Autodesk Inventor part; units mm, degrees
ref_plane "YZ Plane" through (0, 0, 0) normal (1, 0, 0) x (0, 1, 0)
ref_plane "XZ Plane" through (0, 0, 0) normal (0, 1, 0) x (-1, 0, 0)
ref_plane "XY Plane" through (0, 0, 0) normal (0, 0, 1) x (1, 0, 0)
sketch "Sketch1" plane through (0, 0, 0) normal (0, 0, 1) x (1, 0, 0)
  line L0 (0, -12.5) -> (0, 12.5)
  line L1 (9, 12.5) -> (9, -12.5)
  line L2 (9, -12.5) -> (4, -12.5)
  line L3 (4, -12.5) -> (4, 5.5)
  line L4 (4, 5.5) -> (2.5, 5.5)
  line L5 (2.5, 5.5) -> (2.5, 12.5)
  line L6 (2.5, 12.5) -> (9, 12.5)
  point P0 (0, 0)
  point P1 (0, 0)
  dimension "d0" = 18
  dimension "d1" = 25
  dimension "d2" = 8
  dimension "d3" = 5
  dimension "d4" = 18
revolve "Revolution1" add sketch "Sketch1" angle 360 about axis through (0, -12.5, 0) along (0, 1, 0)
sketch "Sketch2" plane through (0, 0, 0) normal (1, 0, 0) x (0, 1, 0)
  line L0 (12.5, -2.5) -> (12.5, 2.5)
  line L1 (-12.5, -4) -> (-12.5, 4)
  point P0 (0, 0)
  point P1 (9, 0)
  point P2 (-9, 0)
  dimension "d6" = 3.5
  dimension "d7" = 3.5
hole "Hole1" at (0, 9, 0) at (0, -9, 0) direction (-1, 0, 0) diameter 3.242 end through all
chamfer "Chamfer1" distance 0.3 angle 45 4 edges at (-9, 12.5, 0) (-2.5, 12.5, 0) (-9, -12.5, 0) (-4, -12.5, 0)
pattern_circular "Circular Pattern1" count 2 over 90 about axis through (0, 0, 0) along (0, 1, 0) of "Hole1"
properties part number "spring-shaft-coupler" material "Aluminum 6061-AHC"
Can you work these out from the model? Positions are in its coordinate system, mm. A direction names the side the tool comes from. Give positions to 0.01 mm unless a question says otherwise; leave off trailing zeros. Loops run counter-clockwise (first coordinate to the right, second up) from the corner with the lowest first, then second, coordinate; pieces in that order, holes last. Notation, with made-up numbers: (70, 43.25) - (90, 43.25) arc R23 ccw to (90, 56.25) - close; hole circle Ø6 at (78.25, -37.5). An arc over 180 degrees is marked (long way). Answer as a JSON object with one key per item and string values.
Q1. If we mould it in two halves opening along X, with no side actions, what happens to faces 1 (the cylindrical face through (1.34, 8.9, -2.11)), 2 (the cylindrical face through (-6.366, -7.562, -0.748)), 3 (the cylindrical face through (4.153, -0.171, -7.985))? For each: pulls with the +X half, pulls with the -X half, needs draft (parallel to the pull), parting line crosses it, or undercut.
Geometry says:
{"face 1": "undercut", "face 2": "needs draft", "face 3": "parting line crosses it"}
Q2. Imagine slicing it at D-D on y = -5. Write out the boundary of the cut face in (x, z).
Geometry says:
{"outline": "circle Ø18 at (0, 0); hole circle Ø8 at (0, 0)"}
Q3. Imagine slicing it at B-B on z = 0. Write out the boundary of the cut face in (x, y), plus the area to 3 significant figures.
Geometry says:
{"outline": "(-9, -12.2) - (-8.7, -12.5) - (-4.3, -12.5) - (-4, -12.2) - (-4, -10.62) - (-9, -10.62) - close; (-9, -7.38) - (-4, -7.38) - (-4, 5.5) - (-2.5, 5.5) - (-2.5, 7.38) - (-9, 7.38) - close; (-9, 10.62) - (-2.5, 10.62) - (-2.5, 12.2) - (-2.8, 12.5) - (-8.7, 12.5) - (-9, 12.2) - close; (2.5, 5.5) - (4, 5.5) - (4, -12.2) - (4.3, -12.5) - (8.7, -12.5) - (9, -12.2) - (9, 12.2) - (8.7, 12.5) - (2.8, 12.5) - (2.5, 12.2) - close", "area": "233 mm²"}
Q4. Will these pins go through, and if not, where does the flat tip stop? P1, Ø1.5, axis at y = -10, z = -4, coming from the -X side; P2, Ø3, axis at x = 0, z = 0, coming from the +Y side; P3, Ø1.5, axis at x = -1, y = 4, coming from the +Z side; P4, Ø1.5, axis at x = 3, y = -6, coming from the -Z side.
Geometry says:
{"P1": "x = -8.39", "P2": "through", "P3": "z = 9", "P4": "z = -8.71"}
Q5. If I drill on L1, parallel to Y at x = 0, z = 4.5; L2, parallel to Z at x = 0, y = 0; L3, parallel to X at y = 4.75, z = -1.5, over which ranges is the centre line in solid material (lowest first)?
Geometry says:
{"L1": "-12.5 to -10.62, -7.38 to 7.38, 10.62 to 12.5", "L2": "-9 to -4, 4 to 9", "L3": "-8.87 to -3.71, 3.71 to 8.87"}
Q6. Which directions (+Z, -Z, +X, -X, +Y, -Y) give clear straight access to the entire face, cutting with the end or side of a thin tool? Please do faces 4 (the cylindrical face through (-5.501, 7.393, 0.211)), 5 (the flat face through (-2.1, 12.5, -2.1)), 6 (the flat face through (2, 5.5, -2)), 7 (the cylindrical face through (-0.748, -7.562, 6.366)), 8 (the flat face through (2, -12.5, -4)).
Geometry says:
{"face 4": "-X", "face 5": "+Z, -Z, +X, -X, +Y", "face 6": "-Y", "face 7": "+Z", "face 8": "+Z, -Z, +X, -X, -Y"}
Q7. Imagine slicing it at A-A on x = 0. Write out the boundary of the cut face in (y, z).
Geometry says:
{"outline": "(-12.5, -8.7) - (-12.2, -9) - (12.2, -9) - (12.5, -8.7) - (12.5, -2.8) - (12.2, -2.5) - (5.5, -2.5) - (5.5, -4) - (-12.2, -4) - (-12.5, -4.3) - close; (-12.5, 4.3) - (-12.2, 4) - (-10.62, 4) - (-10.62, 9) - (-12.2, 9) - (-12.5, 8.7) - close; (-7.38, 4) - (5.5, 4) - (5.5, 2.5) - (7.38, 2.5) - (7.38, 9) - (-7.38, 9) - close; (10.62, 2.5) - (12.2, 2.5) - (12.5, 2.8) - (12.5, 8.7) - (12.2, 9) - (10.62, 9) - close"}
Q8. Imagine slicing it at C-C on y = -9. Write out the boundary of the cut face in (x, z).
Geometry says:
{"outline": "(-8.85, -1.62) arc R9 ccw (long way) to (1.62, 8.85) - (1.62, 3.66) arc R4 cw (long way) to (-3.66, -1.62) - close; (-8.85, 1.62) - (-3.66, 1.62) arc R4 cw to (-1.62, 3.66) - (-1.62, 8.85) arc R9 ccw to start"}
